Geometry check sheet. Reference: the model listing, model coordinates, mm. A direction names the side the tool comes from. Coordinates: 2 decimals unless noted, no trailing zeros. Order: outer loops, then holes, each group sorted by start corner. A loop starts at its lowest first (then second) coordinate and runs counter-clockwise, first axis right, second up. Notation, with made-up numbers: (79, 67) - (133, 67) arc R17 cw to (133, 82) - close; hole circle Ø5 at (-8, 49). An arc over 180 degrees is marked (long way). Return JSON: item names as keys, results as strings. Group by question number.
Item 1: Gauge pin test, flat ends, axial feed: pin 1 (4 mm diameter, centred on x = 5.5, z = 1.5, fed in from +Y); pin 2 (1.6 mm diameter, centred on x = -1, z = 7, fed in from -Y); pin 3 (0.6 mm diameter, centred on x = -0.5, z = 7, fed in from +Y); pin 4 (5 mm diameter, centred on x = 1, y = 2.5, fed in from +Z). Record the tip position at first contact, or that the pin passes through.
Item 2: Section check B-B on y = 0.5. Enter the section's corners in (x, z), then the cut area to 3 significant figures.
Item 3: Section check D-D on x = -4.25. Enter the section's corners in (y, z).
Item 4: Tool access check on faces 1 (the flat face through (6, 0, 7)), 2 (the flat face through (6.5, 0, 2)), 3 (the flat face through (0, -4, 2)), 4 (the flat face through (-6.5, 0, 2)), 5 (the flat face through (3, 4, 7)). Record the directions out of +Z, -Z, +X, -X, +Y, -Y that give a thin tool (end or side, any length) a straight path to the whole face; none if there is none.
Item 5: Section check A-A on x = -6.25. Enter the section's corners in (y, z), then the cut area to 3 significant figures.
Item 6: Section check C-C on z = 2. Enter the section's corners in (x, y), then the cut area to 3 significant figures.
Item 7: Scan lines: probe 1 along X at (y, z) = (2, 0.75); probe 2 along Y at (x, z) = (4.5, 4.75); probe 3 along Z at (x, y) = (-7, 0.75). Record each from-to range of solid material in increasing order.
from build123d import *

# Parameters (mm, degrees)
ESBO_O1_W                = 13
ESBO_O1_H                = 8
RESSALTO_EXTRUS_O1_DEPTH = 5
ESBO_O2_W                = 15
ESBO_O2_H                = 10
RESSALTO_EXTRUS_O2_DEPTH = 1
ESBO_O3_W                = 12
ESBO_O3_H                = 8
RESSALTO_EXTRUS_O3_DEPTH = 2
CORTE_EXTRUS_O1_START    = -8
CORTE_EXTRUS_O1_DEPTH    = 8


# Read off the part's stored shape, not the designer's step: Corte-extrusão1
with BuildPart() as part:
    # Esboço1 → Ressalto-extrusão1 (new body)
    with BuildSketch(Plane.XY):
        Rectangle(ESBO_O1_W, ESBO_O1_H)
    extrude(amount=RESSALTO_EXTRUS_O1_DEPTH)

    # Esboço2 → Ressalto-extrusão2 (add)
    with BuildSketch(Plane.XY.offset(5)):
        Rectangle(ESBO_O2_W, ESBO_O2_H)
    extrude(amount=RESSALTO_EXTRUS_O2_DEPTH)

    # Esboço3 → Ressalto-extrusão3 (add)
    with BuildSketch(Plane.XY.offset(6)):
        Rectangle(ESBO_O3_W, ESBO_O3_H)
    extrude(amount=RESSALTO_EXTRUS_O3_DEPTH)

    # Corte-extrusão1 outline → Corte-extrusão1 (cut)
    with BuildSketch(Plane.XZ.offset(4).offset(CORTE_EXTRUS_O1_START)):
        with BuildLine():
            ThreePointArc((-6, 6), (0.053343774, 6.679937356), (6, 8))
            Line((6, 8), (-6, 8))
            Line((-6, 8), (-6, 6))
        make_face()
    extrude(amount=CORTE_EXTRUS_O1_DEPTH, mode=Mode.SUBTRACT)


solid = part.part
Computed:
{
 "1": {"pin 1": "stops at y = 4", "pin 2": "stops at y = -4", "pin 3": "passes through", "pin 4": "stops at z = 7.36"},
 "2": {"outline": "(-7.5, 5) - (-6.5, 5) - (-6.5, 0) - (6.5, 0) - (6.5, 5) - (7.5, 5) - (7.5, 6) - (6, 6) - (6, 8) arc R57.18 cw to (-6, 6) - (-7.5, 6) - close", "area": "89.4 mm²"},
 "3": {"outline": "(-5, 5) - (-4, 5) - (-4, 0) - (4, 0) - (4, 5) - (5, 5) - (5, 6) - (4, 6) - (4, 6.13) - (-4, 6.13) - (-4, 6) - (-5, 6) - close"},
 "4": {"face 1": "+Z, +X, +Y, -Y", "face 2": "-Z, +X, +Y, -Y", "face 3": "-Z, +X, -X, -Y", "face 4": "-Z, -X, +Y, -Y", "face 5": "+Z, +X, -X, +Y"},
 "5": {"outline": "(-5, 5) - (-4, 5) - (-4, 0) - (4, 0) - (4, 5) - (5, 5) - (5, 6) - (-5, 6) - close", "area": "50.0 mm²"},
 "6": {"outline": "(-6.5, -4) - (6.5, -4) - (6.5, 4) - (-6.5, 4) - close", "area": "104 mm²"},
 "7": {"probe 1": "x = -6.5 to 6.5", "probe 2": "y = -4 to 4", "probe 3": "z = 5 to 6"}
}
